from build123d import *

# Parameters (mm, degrees)
F0_W     = 4
F0_H     = 15
F0_W_2   = 12
F1_DEPTH = 12
F2_DEPTH = 8
F4_DEPTH = 25


with BuildPart() as f1:
    # F0 (on Top) → F1 (new body)
    with BuildSketch(Plane.XY):
        with Locations((-8, 0)):
            Rectangle(F0_W, F0_H)
        Rectangle(F0_W_2, F0_H)
        with Locations((8, 0)):
            Rectangle(F0_W, F0_H)
    extrude(amount=F1_DEPTH)

    # F0 (on Top) → F2 (cut)
    with BuildSketch(Plane.XY):
        Rectangle(F0_W_2, F0_H)
    extrude(amount=F2_DEPTH, mode=Mode.SUBTRACT)

    # F3 (on face) → F4 (join)
    with BuildSketch(Plane.XY.offset(12)):
        Polygon((-10, -7.5), (-10, 7.5), (-15.066023, 7.5), (-15.066023, -7.486796), align=None)
        Polygon((15.066023, 7.5), (10, 7.5), (10, -7.5), (15.066023, -7.486796), align=None)
    extrude(amount=-F4_DEPTH)


solid = f1.part
Check sheet for the modelled part. Datum: model origin and axes. Units: mm. A direction names the side the tool comes from. Round coordinates to 2 decimals unless told otherwise and drop trailing zeros. Order: outer loops, then holes, each group sorted by start corner. A loop starts at its lowest first (then second) coordinate and runs counter-clockwise, first axis right, second up.
(1) Access from +Z, -Z, +X, -X, +Y, -Y to the whole of each face (thin tool, end or side, straight path). Record for faces 1 (the flat face through (7, 7.5, 2)), 2 (the flat face through (0, 0, 8)).
(2) Scan lines: probe 1 along X at (y, z) = (5, 5.5); probe 2 along X at (y, z) = (5, -1.5); probe 3 along Z at (x, y) = (2, -7). Record each from-to range of solid material in increasing order.
(3) Draft check along X on faces 3 (the flat face through (8, 0, 0)), 4 (the flat face through (-13, 0, -13)), 5 (the flat face through (15.066, 0, 0)). Enter one of: pulls with the +X half, pulls with the -X half, needs draft (parallel to the pull), parting line crosses it, or undercut.
(4) Go/stop test with flat-tipped pins: P1, Ø2, axis at x = 8.5, y = -2, coming from the -Z side; P2, Ø6, axis at x = 0.5, y = -2, coming from the -Z side. Record where each tip stops, or that it passes through.
(5) Cross-section at D-D, the plane x = -0.5. Enter the section's corners in (y, z).
(6) Cross-section at B-B, the plane y = -6.25. Enter the section's corners in (x, z).
(7) Cross-section at C-C, the plane z = -8.5. Enter the section's corners in (x, y).
(8) Cross-section at A-A, the plane z = 3.75. Enter the section's corners in (x, y).
Check sheet entries:
1. face 1: +Z, -Z, +X, -X, +Y
1. face 2: -Z, +Y, -Y
2. probe 1: x = -15.07 to -6, 6 to 15.07
2. probe 2: x = -15.07 to -10, 10 to 15.07
2. probe 3: z = 8 to 12
3. face 3: undercut
3. face 4: needs draft
3. face 5: pulls with the +X half
4. P1: stops at z = 0
4. P2: stops at z = 8
5. outline: (-7.5, 8) - (7.5, 8) - (7.5, 12) - (-7.5, 12) - close
6. outline: (-15.07, -13) - (-10, -13) - (-10, 0) - (-6, 0) - (-6, 8) - (6, 8) - (6, 0) - (10, 0) - (10, -13) - (15.07, -13) - (15.07, 12) - (-15.07, 12) - close
7. outline: (-15.07, -7.49) - (-10, -7.5) - (-10, 7.5) - (-15.07, 7.5) - close; (10, -7.5) - (15.07, -7.49) - (15.07, 7.5) - (10, 7.5) - close
8. outline: (-15.07, -7.49) - (-10, -7.5) - (-6, -7.5) - (-6, 7.5) - (-15.07, 7.5) - close; (6, -7.5) - (10, -7.5) - (15.07, -7.49) - (15.07, 7.5) - (6, 7.5) - close
